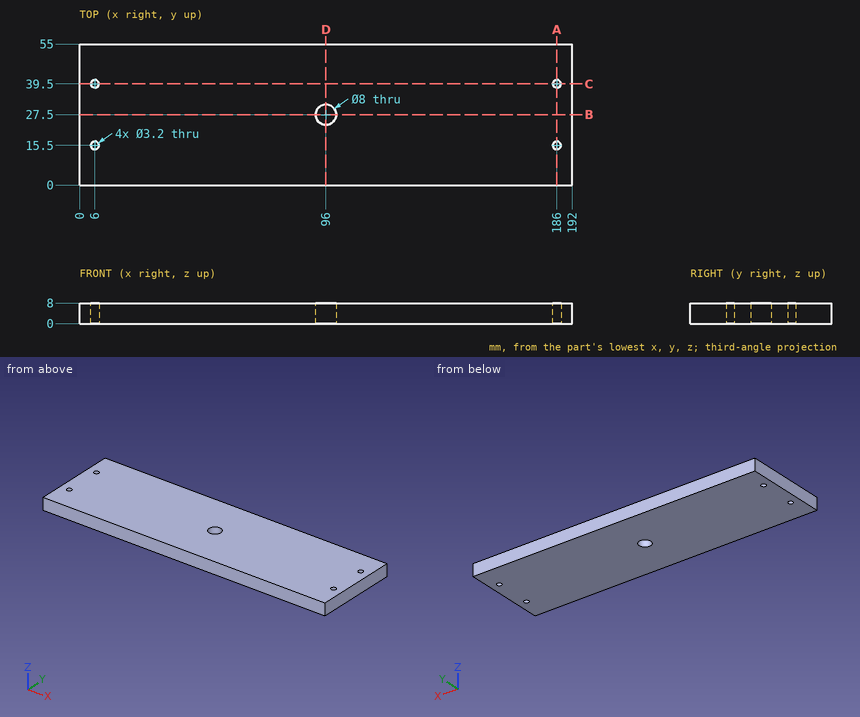
Input: dimensioned drawing with shaded views. Units: mm. Origin: part minimum x, y, z. Coordinates: 2 decimals unless noted, no trailing zeros. Write each loop counter-clockwise with the first axis right and the second up, starting at its lowest first coordinate (ties: lowest second). Pieces come first, ordered by that corner, then holes. Notation, with made-up numbers: M 43.5,2 L 67.5,2 A18 cw 67.5,21 Z; hole C 8.5,-30.75 d5. An arc over 180 degrees is marked long. Answer as a JSON object with one key per item and string values. Group by question number.
(1) Section C-C on y = 39.5. Output: boundary loops of the cut face in (x, z), plus the area to 3 significant figures.
(2) Section D-D on x = 96. Output: boundary loops of the cut face in (y, z), plus the area to 3 significant figures.
(3) Section A-A on x = 186. Output: boundary loops of the cut face in (y, z).
(4) Ray query, line 1 along X through (y, z) = (39.5, 5.5); line 2 along Y through (x, z) = (6, 4.75); line 3 along Y through (x, z) = (96, 5). Return the intervals inside material, ascending. Write a range as [from, to].
(5) Contact query for a flat-ended pin moving along its axis: P1, Ø1.5, axis at x = 143.5, z = 5, coming from the -Y side. Output: stop coordinate, or through.
(6) Section B-B on y = 27.5. Output: boundary loops of the cut face in (x, z).
Result set:
{
 "1": {"outline": "M 0,0 L 4.4,0 L 4.4,8 L 0,8 Z; M 7.6,0 L 184.4,0 L 184.4,8 L 7.6,8 Z; M 187.6,0 L 192,0 L 192,8 L 187.6,8 Z", "area": "1,480 mm2"},
 "2": {"outline": "M 0,0 L 23.5,0 L 23.5,8 L 0,8 Z; M 31.5,0 L 55,0 L 55,8 L 31.5,8 Z", "area": "376 mm2"},
 "3": {"outline": "M 0,0 L 13.9,0 L 13.9,8 L 0,8 Z; M 17.1,0 L 37.9,0 L 37.9,8 L 17.1,8 Z; M 41.1,0 L 55,0 L 55,8 L 41.1,8 Z"},
 "4": {"line 1": "x = [0, 4.4], [7.6, 184.4], [187.6, 192]", "line 2": "y = [0, 13.9], [17.1, 37.9], [41.1, 55]", "line 3": "y = [0, 23.5], [31.5, 55]"},
 "5": {"P1": "stops at y = 0"},
 "6": {"outline": "M 0,0 L 92,0 L 92,8 L 0,8 Z; M 100,0 L 192,0 L 192,8 L 100,8 Z"}
}
